Work out the finished part from the listing and answer in its coordinate system (mm). A direction names the side the tool comes from. Coordinates: 2 decimals unless noted, no trailing zeros. Write each loop counter-clockwise with the first axis right and the second up, starting at its lowest first coordinate (ties: lowest second). Pieces come first, ordered by that corner, then holes. Notation, with made-up numbers: (59, -12.5) - (66, -12.5) arc R19 cw to (66, 13.5) - close; hole circle Ø7 at (65, 4). An arc over 180 degrees is marked (long way). One line per item, written item: value.
```python
from build123d import *

# Parameters (mm, degrees)
F0_W     = 203.2
F0_H     = 50.8
F1_DEPTH = 101.6
F2_R     = 43.460666
F3_DEPTH = 38.1
F4_W     = 82.872769
F4_H     = 50.8
F5_DEPTH = 15.24
F7_DEPTH = 101.6


with BuildPart() as f1:
    # F0 (on Top) → F1 (new body)
    with BuildSketch(Plane.XY):
        with Locations((-13.052889, -64.237624)):
            Rectangle(F0_W, F0_H)
    extrude(amount=F1_DEPTH)

    # F2 (on face) → F3 (join)
    with BuildSketch(Plane.XZ.offset(89.637624)):
        with Locations((-13.052889, 50.8)):
            Circle(F2_R)
    extrude(amount=F3_DEPTH)

    # F4 (on face) → F5 (join)
    with BuildSketch(Plane.XY.offset(101.6)):
        with Locations((-13.317311, -64.237624)):
            Rectangle(F4_W, F4_H)
    extrude(amount=F5_DEPTH)

    # F6 (on face) → F7 (cut)
    with BuildSketch(Plane.YZ.offset(28.119074)):
        Polygon((-89.637624, 116.84), (-89.637624, 101.6), (-64.237624, 116.84), align=None)
    extrude(amount=-F7_DEPTH, mode=Mode.SUBTRACT)


solid = f1.part
```
Item 1: Consider probe 1 along Z at (x, y) = (73, -85.5); probe 2 along Y at (x, z) = (68.5, 9.5); probe 3 along Z at (x, y) = (-46, -85.5). Determine where each line is inside the solid, lowest interval first.
Evaluation:
probe 1: z = 0 to 101.6
probe 2: y = -89.64 to -38.84
probe 3: z = 0 to 104.08
Item 2: Section C-C, the plane x = 19 is taken. Determine the outline of the cut face in (y, z).
Evaluation:
outline: (-127.74, 21.45) - (-89.64, 21.45) - (-89.64, 0) - (-38.84, 0) - (-38.84, 116.84) - (-64.24, 116.84) - (-89.64, 101.6) - (-89.64, 80.15) - (-127.74, 80.15) - close
Item 3: Which of the six approach directions +Z, -Z, +X, -X, +Y, -Y give full straight-line access (tool end or side, diameter ignored) to faces 1 (the face through (-22.47, -108.42, 8.37)), 2 (the face through (-85, -64, 101.6)), 3 (the face through (58, -64, 101.6))?
Evaluation:
face 1: -Y
face 2: +Z, -X, +Y, -Y
face 3: +Z, +X, +Y, -Y
Item 4: Section D-D, the plane x = -22 is taken. Determine the outline of the cut face in (y, z), then the cut area to 3 significant figures.
Evaluation:
outline: (-127.74, 8.27) - (-89.64, 8.27) - (-89.64, 0) - (-38.84, 0) - (-38.84, 116.84) - (-64.24, 116.84) - (-89.64, 101.6) - (-89.64, 93.33) - (-127.74, 93.33) - close
area: 8,980 mm2
Item 5: Given pin 1 (17 mm diameter, centred on y = -74.5, z = 112.5, fed in from -X); pin 2 (7.5 mm diameter, centred on y = -55, z = 107.5, fed in from +X); pin 3 (2 mm diameter, centred on x = 39.5, y = -52, fed in from +Z), each flat-ended and moving along its own axis, determine where each tip first touches the part or whether it passes through.
Evaluation:
pin 1: stops at x = -54.75
pin 2: stops at x = 28.12
pin 3: stops at z = 101.6
Item 6: Section A-A, the plane z = 89.5 is taken. Determine the outline of the cut face in (x, y), then the cut area to 3 significant figures.
Evaluation:
outline: (-114.65, -89.64) - (-32.83, -89.64) - (-32.83, -127.74) - (6.72, -127.74) - (6.72, -89.64) - (88.55, -89.64) - (88.55, -38.84) - (-114.65, -38.84) - close
area: 11,800 mm2
Item 7: Section B-B, the plane y = -80.5 is taken. Determine the outline of the cut face in (x, z), then the cut area to 3 significant figures.
Evaluation:
outline: (-114.65, 0) - (88.55, 0) - (88.55, 101.6) - (28.12, 101.6) - (28.12, 107.08) - (-54.75, 107.08) - (-54.75, 101.6) - (-114.65, 101.6) - close
area: 21,100 mm2
